Geometry: final body of the model. Coordinates: model frame, mm. A direction names the side the tool comes from. Round coordinates to 2 decimals unless told otherwise and drop trailing zeros. Order: outer loops, then holes, each group sorted by start corner. A loop starts at its lowest first (then second) coordinate and runs counter-clockwise, first axis right, second up. Notation, with made-up numbers: (81, 69.5) -> (106, 69.5) arc R11 cw to (106, 75.5) -> close; hole circle Ø11 at (11, 25). An arc over 180 degrees is marked (long way). Put each result on its own line as item: value.
```python
from build123d import *

# Parameters (mm, degrees)
SKETCH1_R           = 13
BOSS_EXTRUDE1_DEPTH = 2
SKETCH2_R           = 4.5
CUT_EXTRUDE1_DEPTH  = 19.493242009
SKETCH3_R           = 1.95
BOSS_EXTRUDE2_DEPTH = 1.4
CHAMFER1_SIZE       = 0.5


with BuildPart() as part:
    # Sketch1 → Boss-Extrude1 (new body)
    with BuildSketch(Plane(origin=(0, 0, 0), x_dir=(1, 0, 0), z_dir=(0, 1, 0))):
        with Locations(Location((0, 0, 0), (0, 0, 270))):
            Circle(SKETCH1_R)
    extrude(amount=BOSS_EXTRUDE1_DEPTH)

    # Sketch2 → Cut-Extrude1 (cut, through all)
    with BuildSketch(Plane(origin=(0, 2, 0), x_dir=(1, 0, 0), z_dir=(0, 1, 0))):
        with Locations(Location((0, 0, 0), (0, 0, 270))):
            Circle(SKETCH2_R)
    extrude(amount=-CUT_EXTRUDE1_DEPTH, mode=Mode.SUBTRACT)

    # Sketch3 → Boss-Extrude2 (add)
    with BuildSketch(Plane(origin=(0, 2, 0), x_dir=(1, 0, 0), z_dir=(0, 1, 0))):
        with Locations(Location((0, 10, 0), (0, 0, 270))):
            Circle(SKETCH3_R)
        with Locations(Location((10, 0, 0), (0, 0, 270))):
            Circle(SKETCH3_R)
        with Locations(Location((-10, 0, 0), (0, 0, 270))):
            Circle(SKETCH3_R)
        with Locations(Location((0, -10, 0), (0, 0, 270))):
            Circle(SKETCH3_R)
    extrude(amount=BOSS_EXTRUDE2_DEPTH)

    # Chamfer1
    chamfer1_edges = [part.edges().sort_by_distance(p)[0] for p in [
        (0, 0, -4.5),
    ]]
    chamfer(chamfer1_edges, length=CHAMFER1_SIZE)


solid = part.part
```
1. Cut plane D-D on x = 5.5. Return loops of the section in (y, z).
Ans:
outline: (0, -11.78) -> (2, -11.78) -> (2, 11.78) -> (0, 11.78) -> close
2. Cut plane B-B on x = 11.25. Return loops of the section in (y, z).
Ans:
outline: (0, -6.51) -> (2, -6.51) -> (2, -1.5) -> (3.4, -1.5) -> (3.4, 1.5) -> (2, 1.5) -> (2, 6.51) -> (0, 6.51) -> close
3. Cut plane A-A on z = 0. Return loops of the section in (x, y).
Ans:
outline: (-13, 0) -> (-5, 0) -> (-4.5, 0.5) -> (-4.5, 2) -> (-8.05, 2) -> (-8.05, 3.4) -> (-11.95, 3.4) -> (-11.95, 2) -> (-13, 2) -> close; (4.5, 0.5) -> (5, 0) -> (13, 0) -> (13, 2) -> (11.95, 2) -> (11.95, 3.4) -> (8.05, 3.4) -> (8.05, 2) -> (4.5, 2) -> close
4. Set-up query: faces 1 (the face through (-8.356, 2.69, 1.048)), 2 (the face through (0, 3.4, -10)). Return all of +Z, -Z, +X, -X, +Y, -Y with unobstructed straight access to the full face (end or side cutting, diameter ignored); none if empty.
Ans:
face 1: +Y
face 2: +Z, -Z, +X, -X, +Y
5. Draft query along Z for faces 3 (the face through (0, 0, 6)), 4 (the face through (8.27, 2.69, 0.9)), 5 (the face through (1.352, 1.26, 4.292)). Return one class per face: +Z half, -Z half, draft (parallel to the pull), parting line (faces both ways), or undercut.
Ans:
face 3: draft
face 4: parting line
face 5: undercut
6. Cut plane C-C on z = -9.75. Return loops of the section in (x, y), and give its area (3 significant figures).
Ans:
outline: (-8.6, 0) -> (8.6, 0) -> (8.6, 2) -> (1.93, 2) -> (1.93, 3.4) -> (-1.93, 3.4) -> (-1.93, 2) -> (-8.6, 2) -> close
area: 39.8 mm²
7. Contact query for flat-ended pins moving along their axis: P1, Ø5, axis at x = 2, z = 0.5, coming from the -Y side; P2, Ø3, axis at x = -1, z = 4.5, coming from the +Y side; P3, Ø1.5, axis at x = 10, y = 3, coming from the -Z side. Output: stop coordinate, or through.
Ans:
P1: y = 0.44
P2: y = 2
P3: z = -1.95
8. Material intervals for probe 1 along X at (y, z) = (1.45, 0); probe 2 along Y at (x, z) = (-5.25, 0.75); probe 3 along Z at (x, y) = (-2, 0.6), sorted ascending.
Ans:
probe 1: -13 to -4.5, 4.5 to 13
probe 2: 0 to 2
probe 3: -12.85 to -4.03, 4.03 to 12.85
